Autodesk Fusion 360 part; units mm, degrees
sketch "Sketch1" plane through (0, 0, 0) normal (0, 0, 1) x (1, 0, 0) in component "Laser Carriage - Motor Side V2"
  line L0 (0, 0) -> (64, 0)
  line L1 (64, 0) -> (64, 120)
  line L2 (64, 120) -> (0, 120)
  line L3 (0, 120) -> (0, 0)
  dimension "d1" = 64
  dimension "d2" = 120
extrude "Extrude1" add sketch "Sketch1" along normal blind 4 in component "Laser Carriage - Motor Side V2"
sketch "Sketch2" plane through (0, 0, 4) normal (0, 0, 1) x (-1, 0, 0) in component "Laser Carriage - Motor Side V2"
  line L0 (0, -120) -> (0, 0)
  line L1 (0, 0) -> (-64, 0)
  line L2 (-64, 0) -> (-64, -120)
  line L3 (-64, -120) -> (0, -120)
  line L4 (-12, -120) -> (-12, 0) construction
  line L5 (-52, -120) -> (-52, 0) construction
  line L6 (0, -12) -> (-64, -12) construction
  line L7 (0, -72) -> (-64, -72) construction
  circle A0 centre (-12, -72) radius 12 construction
  circle A1 centre (-52, -72) radius 12 construction
  circle A2 centre (-12, -72) radius 3
  circle A3 centre (-52, -72) radius 3
  circle A4 centre (-32, -12) radius 12 construction
  circle A5 centre (-32, -12) radius 2.75
  line L8 (0, -85) -> (-64, -85) construction
  line L9 (-32, -85) -> (-32, 0) construction
  line L10 (0, -42) -> (-64, -42) construction
  line L11 (0, -27) -> (-64, -27) construction
  line L12 (0, -56) -> (-64, -56) construction
  line L13 (-21, -56) -> (-21, -27) construction
  line L14 (-43, -56) -> (-43, -27) construction
  line L15 (-21, -56) -> (-43, -56)
  line L16 (-43, -56) -> (-32, -27)
  line L17 (-32, -27) -> (-21, -56)
  point P0 (-32, -42)
  dimension "d8" = 12
  dimension "d13" = 24
  dimension "d14" = 24
  dimension "d16" = 6
  dimension "d17" = 6
  dimension "d40" = 60
  dimension "d53" = 24
  dimension "d55" = 5.5
  dimension "d234" = 13
  dimension "d238" = 20
  dimension "d324" = 30
  dimension "d327" = 20
  dimension "d333" = 15
  dimension "d334" = 56
  dimension "d335" = 11
  dimension "d336" = 11
extrude "Extrude2" cut sketch "Sketch2" against normal up to surface (4 mm away) contours A2 | A3 | A5 | L15 L16 L17 in component "Laser Carriage - Motor Side V2"
sketch "Sketch16" plane through (0, 0, 4) normal (0, 0, 1) x (-1, 0, 0) in component "Laser Carriage - Motor Side V2"
  circle A0 centre (-52, -72) radius 3
  circle A1 centre (-12, -72) radius 3
  line L0 (-64, -120) -> (0, -120)
  line L1 (0, -120) -> (0, 0)
  line L2 (0, 0) -> (-64, 0)
  line L3 (-64, 0) -> (-64, -120)
  circle A2 centre (-32, -12) radius 2.75
  line L4 (0, -91) -> (-64, -91) construction
  line L5 (-64, -120) -> (0, -120) construction
  line L6 (-6, 0) -> (-6, -120) construction
  line L7 (0, -120) -> (0, 0) construction
  line L8 (-58, 0) -> (-58, -120) construction
  circle A3 centre (-6, -91) radius 4
  circle A4 centre (-58, -91) radius 4
  line L9 (0, 0) -> (-64, 0)
  line L10 (-43, -56) -> (-32, -27)
  line L11 (-32, -27) -> (-21, -56)
  line L12 (-21, -56) -> (-43, -56)
  dimension "d268" = 6
  dimension "d269" = 6
  dimension "d270" = 8
  dimension "d271" = 8
  dimension "d273" = 91
extrude "Extrude17" cut sketch "Sketch16" against normal up to surface (4 mm away) contours A3 | A4 in component "Laser Carriage - Motor Side V2"
sketch "Sketch18" plane through (0, 0, 4) normal (0, 0, 1) x (-1, 0, 0) in component "Laser Carriage - Motor Side V2"
  line L0 (-64, -120) -> (0, -120)
  line L1 (-32, -120) -> (-32, 0) construction
  line L2 (0, 0) -> (-64, 0) construction
  line L3 (-47.5, -120) -> (-47.5, 0) construction
  line L4 (-16.5, 0) -> (-16.5, -120) construction
  line L5 (-2, -113.5) -> (-62, -113.5) construction
  line L6 (-2, -82.5) -> (-62, -82.5) construction
  line L7 (-2, -98) -> (-62, -98) construction
  circle A0 centre (-32, -98) radius 11.5
  circle A1 centre (-16.5, -113.5) radius 1.65
  circle A2 centre (-47.5, -113.5) radius 1.65
  circle A3 centre (-16.5, -82.5) radius 1.65
  circle A4 centre (-47.5, -82.5) radius 1.65
  line L8 (-2, -120) -> (-62, -120) construction
  line L9 (-54, -120) -> (-10, -120) construction
  line L10 (-10, -120) -> (-10, -76) construction
  line L11 (-10, -76) -> (-54, -76) construction
  line L12 (-54, -76) -> (-54, -120) construction
  line L13 (-54, -120) -> (-10, -76) construction
  line L14 (-10, -120) -> (-54, -76) construction
  point P0 (-32, -98)
  dimension "d275" = 15.5
  dimension "d276" = 15.5
  dimension "d279" = 98
  dimension "d280" = 15.5
  dimension "d281" = 15.5
  dimension "d283" = 23
  dimension "d284" = 3.3
  dimension "d285" = 3.3
  dimension "d286" = 3.3
  dimension "d287" = 3.3
  dimension "d288" = 6.5
  dimension "d289" = 44
  dimension "d290" = 44
extrude "Extrude18" cut sketch "Sketch18" against normal up to surface (4 mm away) in component "Laser Carriage - Motor Side V2"
sketch "Sketch20" plane through (0, 0, 0) normal (0, 0, -1) x (1, 0, 0) in component "Laser Carriage - Motor Side V2"
  circle A0 centre (16.5, -113.5) radius 1.65
  circle A1 centre (47.5, -113.5) radius 1.65
  circle A2 centre (16.5, -82.5) radius 1.65
  circle A3 centre (32, -98) radius 11.5
  circle A4 centre (47.5, -82.5) radius 1.65
  circle A5 centre (6, -91) radius 4
  circle A6 centre (58, -91) radius 4
  circle A7 centre (52, -72) radius 3
  circle A8 centre (32, -12) radius 2.75
  circle A9 centre (12, -72) radius 3
  line L0 (0, 0) -> (0, -120)
  line L1 (0, -120) -> (64, -120)
  line L2 (64, -120) -> (64, 0)
  line L3 (64, 0) -> (0, 0)
  line L4 (64, -120) -> (64, -148)
  line L5 (32, -120) -> (32, -148)
  line L6 (32, -148) -> (64, -148)
  line L7 (32, -27) -> (43, -56)
  line L8 (43, -56) -> (21, -56)
  line L9 (21, -56) -> (32, -27)
  dimension "d303" = 28
  dimension "d304" = 28
extrude "Extrude20" add sketch "Sketch20" against normal blind 4 contours L1 L4 L5 L6 in component "Laser Carriage - Motor Side V2"
sketch "Sketch21" plane through (0, 0, 4) normal (0, 0, 1) x (-1, 0, 0) in component "Laser Carriage - Motor Side V2"
  circle A0 centre (-16.5, -113.5) radius 1.65
  circle A1 centre (-47.5, -113.5) radius 1.65
  circle A2 centre (-16.5, -82.5) radius 1.65
  circle A3 centre (-32, -98) radius 11.5
  circle A4 centre (-47.5, -82.5) radius 1.65
  circle A5 centre (-6, -91) radius 4
  circle A6 centre (-58, -91) radius 4
  line L0 (0, -120) -> (0, 0)
  line L1 (0, 0) -> (-64, 0)
  line L2 (-64, 0) -> (-64, -148)
  line L3 (-64, -148) -> (-32, -148)
  line L4 (-32, -148) -> (-32, -120)
  line L5 (-32, -120) -> (0, -120)
  circle A7 centre (-52, -72) radius 3
  circle A8 centre (-32, -12) radius 2.75
  circle A9 centre (-12, -72) radius 3
  line L6 (-48, -148) -> (-48, -122) construction
  line L7 (-32, -138) -> (-64, -138) construction
  line L8 (-54, -120) -> (-10, -120) construction
  line L9 (-32, -143) -> (-64, -143) construction
  line L10 (-53, -148) -> (-53, -138) construction
  line L11 (-43, -148) -> (-43, -138) construction
  circle A10 centre (-43, -143) radius 2.05
  circle A11 centre (-53, -143) radius 2.05
  line L12 (-43, -56) -> (-32, -27)
  line L13 (-32, -27) -> (-21, -56)
  line L14 (-21, -56) -> (-43, -56)
  dimension "d309" = 18
  dimension "d310" = 5
  dimension "d311" = 10
  dimension "d312" = 5
  dimension "d313" = 4.1
  dimension "d314" = 4.1
extrude "Extrude21" cut sketch "Sketch21" against normal blind 4 contours A10 | A11 in component "Laser Carriage - Motor Side V2"
sketch "Sketch22" plane through (0, 0, 4) normal (0, 0, 1) x (-1, 0, 0) in component "Laser Carriage - Motor Side V2"
  circle A0 centre (-43, -143) radius 2.05
  circle A1 centre (-53, -143) radius 2.05
  circle A2 centre (-16.5, -113.5) radius 1.65
  circle A3 centre (-47.5, -113.5) radius 1.65
  circle A4 centre (-16.5, -82.5) radius 1.65
  circle A5 centre (-32, -98) radius 11.5
  circle A6 centre (-47.5, -82.5) radius 1.65
  circle A7 centre (-6, -91) radius 4
  circle A8 centre (-58, -91) radius 4
  circle A9 centre (-12, -72) radius 3
  circle A10 centre (-52, -72) radius 3
  circle A11 centre (-32, -12) radius 2.75
  line L0 (0, -120) -> (0, 0)
  line L1 (0, 0) -> (-64, 0)
  line L2 (-64, 0) -> (-64, -148)
  line L3 (-64, -148) -> (-32, -148)
  line L4 (-32, -148) -> (-32, -120)
  line L5 (-32, -120) -> (0, -120)
  circle A12 centre (-12, -72) radius 12
  circle A13 centre (-52, -72) radius 12
  circle A14 centre (-32, -12) radius 12
  line L6 (-0.6158, -68.2053) -> (-20.6158, -8.2053)
  line L7 (-63.3842, -68.2053) -> (-43.3842, -8.2053)
  line L8 (-43, -56) -> (-32, -27)
  line L9 (-32, -27) -> (-21, -56)
  line L10 (-21, -56) -> (-43, -56)
  dimension "d328" = 24
  dimension "d329" = 24
  dimension "d330" = 24
extrude "Extrude22" cut sketch "Sketch22" against normal up to surface (4 mm away) contours L0 L1 A12 A14 L6 | L1 L2 A13 A14 L7 in component "Laser Carriage - Motor Side V2"
sketch "Sketch23" plane through (0, 0, 4) normal (0, 0, 1) x (-1, 0, 0) in component "Laser Carriage - Motor Side V2"
  arc A0 (-63.3842, -68.2053) -> (-64, -72) centre (-52, -72) ccw
  line L0 (-64, -72) -> (-64, -148)
  line L1 (-64, -148) -> (-32, -148)
  line L2 (-32, -148) -> (-32, -120)
  line L3 (-32, -120) -> (0, -120)
  line L4 (0, -120) -> (0, -72)
  arc A1 (0, -72) -> (-0.6158, -68.2053) centre (-12, -72) ccw
  line L5 (-0.6158, -68.2053) -> (-20.6158, -8.2053)
  arc A2 (-20.6158, -8.2053) -> (-43.3842, -8.2053) centre (-32, -12) ccw
  line L6 (-43.3842, -8.2053) -> (-63.3842, -68.2053)
  circle A3 centre (-43, -143) radius 2.05
  circle A4 centre (-53, -143) radius 2.05
  circle A5 centre (-16.5, -113.5) radius 1.65
  circle A6 centre (-47.5, -113.5) radius 1.65
  circle A7 centre (-16.5, -82.5) radius 1.65
  circle A8 centre (-32, -98) radius 11.5
  circle A9 centre (-47.5, -82.5) radius 1.65
  circle A10 centre (-6, -91) radius 4
  circle A11 centre (-58, -91) radius 4
  circle A12 centre (-12, -72) radius 3
  circle A13 centre (-52, -72) radius 3
  circle A14 centre (-32, -12) radius 2.75
  line L7 (-43, -56) -> (-32, -27)
  line L8 (-32, -27) -> (-21, -56)
  line L9 (-21, -56) -> (-43, -56)
fillet "Fillet11" radius 5 1 edges at (32, 120, 2) in component "Laser Carriage - Motor Side V2"
fillet "Fillet11" radius 2 2 edges at (32, 148, 2) (64, 148, 2) in component "Laser Carriage - Motor Side V2"
fillet "Fillet11" radius 2 3 edges at (21, 56, 2) (43, 56, 2) (32, 27, 2) in component "Laser Carriage - Motor Side V2"
fillet "Fillet11" radius 10 1 edges at (0, 120, 2) in component "Laser Carriage - Motor Side V2"
component "Laser Carriage - Motor Side V2" placed x (1, 0, 0) y (0, 1, 0) z (0, 0, 1) at (0, 0, 0)
Work out the finished part from the listing and answer in its coordinate system (mm). A direction names the side the tool comes from. Give positions to 0.01 mm unless a question says otherwise; leave off trailing zeros. Order: outer loops, then holes, each group sorted by start corner. A loop starts at its lowest first (then second) coordinate and runs counter-clockwise, first axis right, second up.
1. Section B-B, the plane z = 3 is taken. Give the number of separate pieces and of enclosed holes in the cut face, and give its area (3 significant figures).
Result sheet:
separate pieces: 1
enclosed holes: 13
area: 5,930 mm2
2. Each of these flat-tipped pins is pushed along its axis until it touches: P1, Ø2, axis at y = 35, z = 2.5, coming from the +X side; P2, Ø1, axis at y = 24.5, z = 1, coming from the -X side. Where does it stop, or does it pass through?
Result sheet:
P1: stops at x = 52.65
P2: stops at x = 15.02
3. Straight lines are drawn through the part: L1, parallel to X at y = 82.5, z = 1.35; L2, parallel to X at y = 143, z = 2.85; L3, parallel to X at y = 11.5, z = 2.5. For each, find the intervals that lie inside material, in ascending order.
Result sheet:
L1: x = 0 to 14.85, 18.15 to 45.85, 49.15 to 64
L2: x = 32 to 40.95, 45.05 to 50.95, 55.05 to 64
L3: x = 19.52 to 29.3, 34.7 to 44.48
4. The mould has two halves that part along X. Classify faces 3 (the flat face through (37.98, 42.76, 2.03)), 4 (the flat face through (48, 148, 2)), 5 (the flat face through (53.524, 38.625, 2.028)): released by +X, released by -X, zero draft, split by the parting line, or undercut.
Result sheet:
face 3: undercut
face 4: zero draft
face 5: released by +X
5. Section A-A, the plane y = 143 is taken. Determine the outline of the cut face in (x, z), and give its area (3 significant figures).
Result sheet:
outline: (32, 0) - (40.95, 0) - (40.95, 4) - (32, 4) - close; (45.05, 0) - (50.95, 0) - (50.95, 4) - (45.05, 4) - close; (55.05, 0) - (64, 0) - (64, 4) - (55.05, 4) - close
area: 95.2 mm2
6. For faces 1 (the cylindrical face through (32, 0, 2)), 2 (the cylindrical face through (22.236, 55.114, 1.972)), determine the directions among +Z, -Z, +X, -X, +Y, -Y from which every point of the face is accessible in a straight line to the end or side of a thin tool.
Result sheet:
face 1: +Z, -Z, -Y
face 2: +Z, -Z
7. Section D-D, the plane x = 6 is taken. Determine the outline of the cut face in (y, z), and give its area (3 significant figures).
Result sheet:
outline: (52.05, 0) - (87, 0) - (87, 4) - (52.05, 4) - close; (95, 0) - (119.17, 0) - (119.17, 4) - (95, 4) - close
area: 236 mm2
8. Section C-C, the plane y = 98 is taken. Determine the outline of the cut face in (x, z), and give its area (3 significant figures).
Result sheet:
outline: (0, 0) - (20.5, 0) - (20.5, 4) - (0, 4) - close; (43.5, 0) - (64, 0) - (64, 4) - (43.5, 4) - close
area: 164 mm2
